The listing builds one solid part. Answer for the finished solid, in the listing's coordinates (mm). Face numbers are marked on the shaded views. A direction names the side the tool comes from. Coordinates: 2 decimals unless noted, no trailing zeros. Order: outer loops, then holes, each group sorted by start corner. A loop starts at its lowest first (then second) coordinate and runs counter-clockwise, first axis right, second up. Notation, with made-up numbers: (69, 58) - (97, 58) arc R13 cw to (97, 80) - close; hole circle Ø9 at (76.25, 14.5). An arc over 180 degrees is marked (long way). Use a Markdown table: item, result. Add a question column.
Item 1: The mould has two halves that part along X. Classify the marked faces 3 and 4: released by +X, released by -X, zero draft, split by the parting line, or undercut.
Item 2: The part is cut by section B-B, the plane z = 3. Give the vertices of the cut face in (x, y).
Item 3: The part is cut by section D-D, the plane z = -2. Give the vertices of the cut face in (x, y), then the cut area to 3 significant figures.
Item 4: Find the intervals of material crossed by line 1 along Z through (x, y) = (19.05, -1.1); line 2 along X through (y, z) = (5, 0.25); line 3 along Z through (x, y) = (-19.05, -1.1), in increasing order.
Item 5: The part is cut by section A-A, the plane x = -11.43. Give the vertices of the cut face in (y, z).
Item 6: For the marked faces 1 and 2, determine the directions among +Z, -Z, +X, -X, +Y, -Y from which every point of the face is accessible in a straight line to the end or side of a thin tool.
Item 7: The part is cut by section C-C, the plane y = 7.5. Give the vertices of the cut face in (x, z), then the cut area to 3 significant figures.
Item 8: Flat-ended cylindrical pins translate along their axes: P1, Ø8, axis at y = 5.5, z = 7.5, coming from the +X side; P2, Ø2.5, axis at x = -19.05, z = 7.493, coming from the +Y side; P3, Ø2, axis at x = 14.5, y = 3, coming from the +Z side. Find the tip coordinate at first contact, or state that the pin passes through.
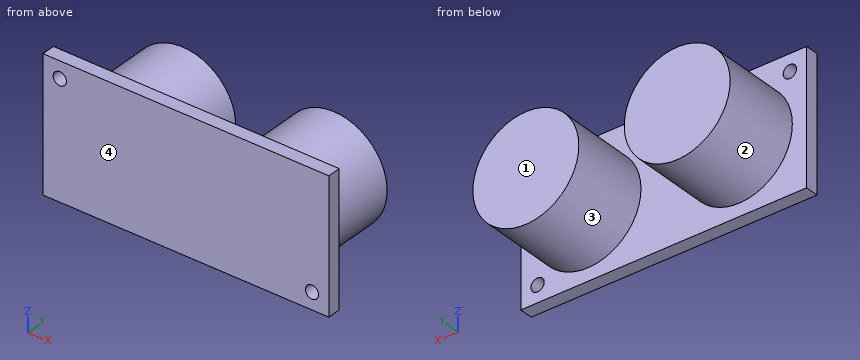
from build123d import *

# Parameters (mm, degrees)
F0_W     = 43.18
F0_H     = 20.066
F1_DEPTH = 2
F3_D     = 2
F4_R     = 8
F5_DEPTH = 12


with BuildPart() as f1:
    # F0 (on Front) → F1 (new body)
    with BuildSketch(Plane.XZ):
        Rectangle(F0_W, F0_H)
    extrude(amount=F1_DEPTH)

    # F3 (through all)
    with Locations(Plane.XZ.offset(2)):
        with Locations((-19.05, 7.493), (19.05, -7.493)):
            Hole(F3_D / 2)

    # F4 (on face) → F5 (join)
    with BuildSketch(Plane(origin=(0, 0, 0), x_dir=(-1, 0, 0), z_dir=(0, 1, 0))):
        with Locations((11.43, -0.127)):
            Circle(F4_R)
        with Locations((-11.43, -0.127)):
            Circle(F4_R)
    extrude(amount=F5_DEPTH)


solid = f1.part
Solution:
| question | item | result |
|---|---|---|
| 1 | face 3 | undercut |
| 1 | face 4 | zero draft |
| 2 | outline | (-21.59, -2) - (21.59, -2) - (21.59, 0) - (18.79, 0) - (18.79, 12) - (4.07, 12) - (4.07, 0) - (-4.07, 0) - (-4.07, 12) - (-18.79, 12) - (-18.79, 0) - (-21.59, 0) - close |
| 3 | outline | (-21.59, -2) - (21.59, -2) - (21.59, 0) - (19.21, 0) - (19.21, 12) - (3.65, 12) - (3.65, 0) - (-3.65, 0) - (-3.65, 12) - (-19.21, 12) - (-19.21, 0) - (-21.59, 0) - close |
| 3 | area | 460 mm2 |
| 4 | line 1 | z = -10.03 to -8.49, -6.49 to 10.03 |
| 4 | line 2 | x = -19.42 to -3.44, 3.44 to 19.42 |
| 4 | line 3 | z = -10.03 to 6.49, 8.49 to 10.03 |
| 5 | outline | (-2, -10.03) - (0, -10.03) - (0, -8.13) - (12, -8.13) - (12, 7.87) - (0, 7.87) - (0, 10.03) - (-2, 10.03) - close |
| 6 | face 1 | +Z, -Z, +X, -X, +Y |
| 6 | face 2 | +Y |
| 7 | outline | circle Ø16 at (-11.43, -0.13); circle Ø16 at (11.43, -0.13) |
| 7 | area | 402 mm2 |
| 8 | P1 | stops at x = 18.56 |
| 8 | P2 | stops at y = 0 |
| 8 | P3 | stops at z = 7.6 |
